from build123d import *

# Parameters (mm, degrees)
BOSS_EXTRUDE1_DEPTH = 238
SKETCH3_W           = 15
SKETCH3_H           = 15
CUT_EXTRUDE1_DEPTH  = 54


with BuildPart() as part:
    # Sketch2 → Boss-Extrude1 (new body)
    with BuildSketch(Plane.XY.offset(-3)):
        with BuildLine():
            Line((446.391965645, 20.11245238), (474.43313548, 20.11245238))
            Line((474.43313548, 20.11245238), (447.390900992, 27.530319971))
            ThreePointArc((447.390900992, 27.530319971), (442.649552271, 24.39262378), (446.391965645, 20.11245238))
        make_face()
    extrude(amount=BOSS_EXTRUDE1_DEPTH)

    # Sketch3 → Cut-Extrude1 (cut)
    with BuildSketch(Plane.XZ.offset(30.589717262)):
        with Locations((450.115770482, 182.5)):
            Rectangle(SKETCH3_W, SKETCH3_H)
        with Locations((450.115770482, 49.5)):
            Rectangle(SKETCH3_W, SKETCH3_H)
    extrude(amount=-CUT_EXTRUDE1_DEPTH, mode=Mode.SUBTRACT)


solid = part.part
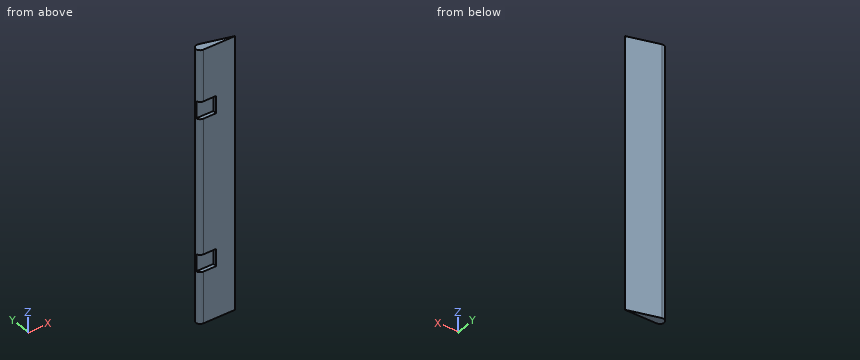
Can you work these out from the model? Positions are in its coordinate system, mm. Give positions to 0.01 mm unless a question says otherwise; leave off trailing zeros. Order: outer loops, then holes, each group sorted by start corner. A loop starts at its lowest first (then second) coordinate and runs counter-clockwise, first axis right, second up. Notation, with made-up numbers: M 33,-10 L 59,-10 A32 ccw 59,24 Z; hole C 65,85 d9. An arc over 180 degrees is marked long. One line per item, written item: value.
Item 1: If we section it at B-B on y = 21.25: Write out the boundary of the cut face in (x, z).
Verdict:
outline: M 443.69,-3 L 470.29,-3 L 470.29,235 L 443.69,235 L 443.69,190 L 457.62,190 L 457.62,175 L 443.69,175 L 443.69,57 L 457.62,57 L 457.62,42 L 443.69,42 Z
Item 2: If we section it at D-D on x = 460: Write out the boundary of the cut face in (y, z), and give its area (3 significant figures).
Verdict:
outline: M 20.11,-3 L 24.07,-3 L 24.07,235 L 20.11,235 Z
area: 942 mm2
Item 3: Please list where these lines run through material, in increasing order: line 1 (Z direction, x = 449, y = 21); line 2 (Y direction, x = 448, z = 142.5); line 3 (Y direction, x = 446, z = 70.5).
Verdict:
line 1: -3 to 42, 57 to 175, 190 to 235
line 2: 20.11 to 27.36
line 3: 20.13 to 27.64
Item 4: If we section it at C-C on z = 69: Write out the boundary of the cut face in (x, y), and give its area (3 significant figures).
Verdict:
outline: M 446.39,20.11 L 474.43,20.11 L 447.39,27.53 A3.78 ccw long Z
area: 130 mm2
Item 5: If we section it at A-A on x = 449.5: Write out the boundary of the cut face in (y, z), and give its area (3 significant figures).
Verdict:
outline: M 20.11,-3 L 26.95,-3 L 26.95,235 L 20.11,235 L 20.11,190 L 23.41,190 L 23.41,175 L 20.11,175 L 20.11,57 L 23.41,57 L 23.41,42 L 20.11,42 Z
area: 1,530 mm2
Item 6: For pin 1 (1.6 mm diameter, centred on y = 22, z = 183.5, fed in from -X); pin 2 (4.5 mm diameter, centred on x = 451.5, z = 51.5, fed in from -Y), each with a flat end and sliding along its axis, tell me the tip position at first contact or that it passes through.
Verdict:
pin 1: x = 457.62
pin 2: y = 23.41
